Autodesk Inventor part; units mm, degrees
ref_plane "YZ Plane" through (0, 0, 0) normal (1, 0, 0) x (0, 1, 0)
ref_plane "XZ Plane" through (0, 0, 0) normal (0, 1, 0) x (-1, 0, 0)
ref_plane "XY Plane" through (0, 0, 0) normal (0, 0, 1) x (1, 0, 0)
sketch "Sketch1" plane through (0, 0, 0) normal (0, 0, 1) x (1, 0, 0)
  circle A0 centre (775, 48) radius 5
  circle A1 centre (0, 0) radius 5
  line L0 (0, 0) -> (611.8616, 0) construction
  line L1 (0, -10) -> (611.8616, -10)
  line L2 (611.8616, 10) -> (0, 10)
  arc A2 (0, 10) -> (0, -10) centre (0, 0) ccw
  arc A3 (611.8616, -10) -> (611.8616, 10) centre (611.8616, 0) ccw
  line L3 (611.8616, 0) -> (695, 48) construction
  line L4 (616.8616, -8.6603) -> (700, 39.3397)
  line L5 (690, 56.6603) -> (606.8616, 8.6603)
  arc A4 (606.8616, 8.6603) -> (616.8616, -8.6603) centre (611.8616, 0) ccw
  arc A5 (700, 39.3397) -> (690, 56.6603) centre (695, 48) ccw
  line L6 (695, 48) -> (775, 48) construction
  line L7 (695, 38) -> (775, 38)
  line L8 (775, 58) -> (695, 58)
  arc A6 (695, 58) -> (695, 38) centre (695, 48) ccw
  arc A7 (775, 38) -> (775, 58) centre (775, 48) ccw
  point P0 (305.9308, 0)
  point P1 (653.4308, 24)
  point P2 (735, 48)
  point P3 (616.8616, -8.6603)
  point P4 (697.6795, 38)
  point P5 (609.1821, 10)
  dimension "d0" = 775
  dimension "d1" = 10
  dimension "d2" = 48
  dimension "d4" = 10
  dimension "d5" = 30
  dimension "d6" = 80
extrude "Extrusion1" add sketch "Sketch1" along normal blind 6
fillet "Fillet1" radius 10 2 edges at (697.6795, 38, 3) (609.1821, 10, 3)
properties part number "FRC001-1"
Work out the finished part from the listing and answer in its coordinate system (mm). Give positions to 0.01 mm unless a question says otherwise; leave off trailing zeros. Order: outer loops, then holes, each group sorted by start corner. A loop starts at its lowest first (then second) coordinate and runs counter-clockwise, first axis right, second up. Notation, with made-up numbers: (48.5, -8) - (94.5, -8) arc R18 ccw to (94.5, 11) - close; hole circle Ø8 at (-18.5, -34.75). An arc over 180 degrees is marked (long way). Answer as CSV lines item,"result". Start each with the question number.
Q1. The part is cut by section B-B (x = 371). Write down the section's boundary in (y, z), then the cut area to 3 significant figures.
Q2. The part is cut by section C-C (y = 19.5). Write down the section's boundary in (x, z), then the cut area to 3 significant figures.
Q3. Given pin 1 Ø2 at (x, z) = (662.5, 1) entering from -Y; pin 2 Ø3 at (x, z) = (400, 2) entering from +Y; pin 3 Ø3 at (y, z) = (33.5, 1) entering from +X; pin 4 Ø10 at (x, y) = (245, 1) entering from -Z, each flat-ended and moving along its own axis, determine where each tip first touches the part or whether it passes through.
Q4. The part is cut by section A-A (z = 1.95). Write down the section's boundary in (x, y), then the cut area to 3 significant figures.
Q5. Find the intervals of material crossed by L1, parallel to Y at x = 0, z = 1.45; L2, parallel to Y at x = 775, z = 3.85; L3, parallel to X at y = 44.5, z = 3.9, in increasing order. Write a range as [from, to].
Check result:
1,outline,"(-10, 0) - (10, 0) - (10, 6) - (-10, 6) - close"
1,area,"120 mm²"
2,outline,"(625.64, 0) - (665.64, 0) - (665.64, 6) - (625.64, 6) - close"
2,area,"240 mm²"
3,pin 1,"stops at y = 17.11"
3,pin 2,"stops at y = 10"
3,pin 3,"stops at x = 692.48"
3,pin 4,"stops at z = 0"
4,outline,"(0, -10) - (611.86, -10) arc R10 ccw to (616.86, -8.66) - (695.36, 36.66) arc R10 cw to (700.36, 38) - (775, 38) arc R10 ccw to (775, 58) - (695, 58) arc R10 ccw to (690, 56.66) - (611.5, 11.34) arc R10 cw to (606.5, 10) - (0, 10) arc R10 ccw to start; hole circle Ø10 at (0, 0); hole circle Ø10 at (775, 48)"
4,area,"15,900 mm²"
5,L1,"y = [-10, -5], [5, 10]"
5,L2,"y = [38, 43], [53, 58]"
5,L3,"x = [668.94, 771.43], [778.57, 784.37]"
